Geometry: see drawing. Coordinates: mm, zero at the bounding-box minimum. Coordinates: 2 decimals unless noted, no trailing zeros. Order: outer loops, then holes, each group sorted by start corner. A loop starts at its lowest first (then second) coordinate and runs counter-clockwise, first axis right, second up.
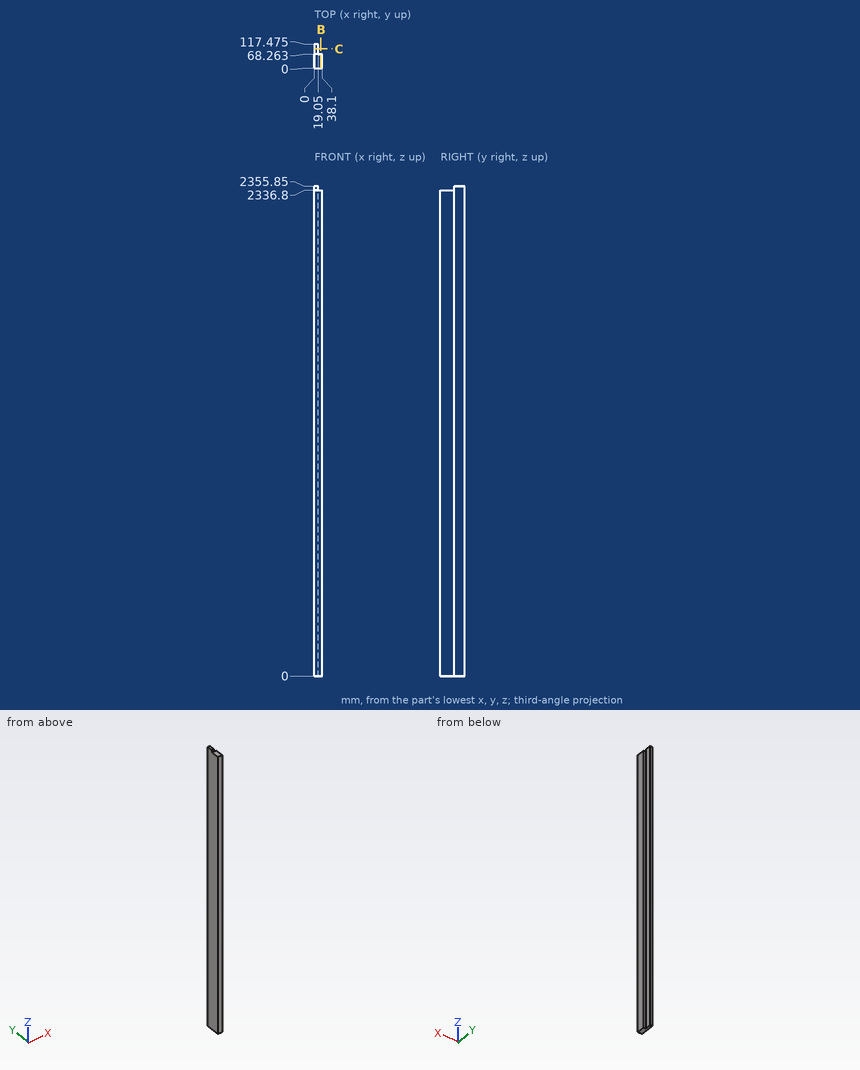
Item 1: Ray query, probe 1 along Z at (x, y) = (22, 68); probe 2 along Y at (x, z) = (21.5, 1318.5); probe 3 along X at (y, z) = (81, 375.5). Return the intervals inside material, ascending.
Response values:
probe 1: z = 0 to 2336.8
probe 2: y = 0 to 68.26
probe 3: x = 0 to 19.05
Item 2: Cut plane B-B on x = 32. Return loops of the section in (y, z), then the cut area to 3 significant figures.
Response values:
outline: (0, 0) - (68.26, 0) - (68.26, 2336.8) - (0, 2336.8) - close
area: 160,000 mm2
Item 3: Pin query (flat end, axial travel): pin 1 Ø5.5 at (x, z) = (8, 2342) entering from -Y; pin 2 Ø11.5 at (x, y) = (15.5, 36.5) entering from +Z; pin 3 Ø21 at (x, z) = (33.5, 1108) entering from +Y. Return the tip coordinate at first contact, or that it passes through.
Response values:
pin 1: stops at y = 68.26
pin 2: stops at z = 2336.8
pin 3: stops at y = 68.26
Item 4: Cut plane C-C on y = 94. Return loops of the section in (x, z), then the cut area to 3 significant figures.
Response values:
outline: (0, 0) - (19.05, 0) - (19.05, 2355.85) - (0, 2355.85) - close
area: 44,900 mm2
